Part model, mm, in its own coordinate system. Coordinates: 2 decimals unless noted, no trailing zeros. Loops run counter-clockwise (first coordinate to the right, second up) from the corner with the lowest first, then second, coordinate; pieces in that order, holes last. Notation, with made-up numbers: (-34, -34.5) -> (-3, -34.5) arc R8 cw to (-3, -26.5) -> close; hole circle Ø7 at (-11, 79.25). An arc over 180 degrees is marked (long way). One line per question, with ' | ' between items. Start each with the question number.
1) Cut at A-A (x = 75). List the corners of the cut face in (y, z), plus the area to 3 significant figures.
2) Cut at C-C (z = 53). List the corners of the cut face in (x, y).
3) Cut at B-B (z = -399.5). List the corners of the cut face in (x, y).
4) Probe L1, parallel to Y at x = 64, z = -62; L2, parallel to Y at x = 82, z = -1046. List the from-to ranges inside material, lowest first. Write a range as from..to.
5) Drop flat-ended pins along their axis: pin 1 (6 mm diameter, centred on x = 56.5, y = 4, fed in from -Z); pin 2 (8 mm diameter, centred on x = 34, z = 36, fed in from +Y); pin 3 (4 mm diameter, centred on x = 45, y = 24, fed in from -Z). Give the stop position or say it passes through.
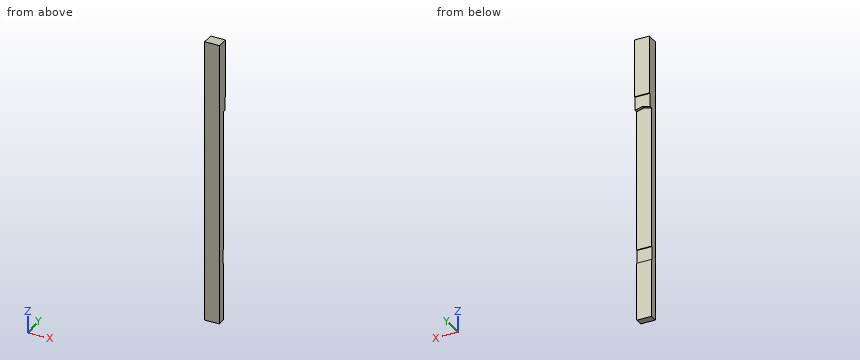
Autodesk Inventor part; units mm, degrees
ref_plane "YZ Plane" through (0, 0, 0) normal (1, 0, 0) x (0, 1, 0)
ref_plane "XZ Plane" through (0, 0, 0) normal (0, 1, 0) x (-1, 0, 0)
ref_plane "XY Plane" through (0, 0, 0) normal (0, 0, 1) x (1, 0, 0)
sketch "Эскиз1" plane through (0, 0, 0) normal (1, 0, 0) x (0, 1, 0)
  line L0 (0, 0) -> (0, -970)
  line L1 (0, -970) -> (-5, -970)
  line L2 (-5, -970) -> (-5, -1063)
  line L3 (-5, -1063) -> (0, -1063)
  line L4 (0, -1063) -> (0, -1463)
  line L5 (0, -1463) -> (-50, -1463)
  line L6 (-50, -1463) -> (-50, 493)
  line L7 (0, 0) -> (21, 0)
  line L8 (21, 0) -> (21, 93)
  line L9 (21, 93) -> (26, 93)
  line L10 (26, 93) -> (26, 493)
  line L11 (26, 493) -> (-50, 493)
  dimension "d0" = 970
  dimension "d1" = 5
  dimension "d2" = 93
  dimension "d3" = 400
  dimension "d4" = 50
  dimension "d5" = 21
  dimension "d6" = 93
  dimension "d7" = 5
  dimension "d8" = 400
  dimension "d9" = 1956
extrude "Выдавливание1" add sketch "Эскиз1" along normal blind 100
sketch "Эскиз2" plane through (0, 21, 93) normal (0, 1, 0) x (1, 0, 0)
  line L0 (0, 91.3764) -> (49.9516, 78.389)
  line L1 (0, 93) -> (0, 91.3764)
  line L2 (0, 93) -> (99.9032, 93)
  line L3 (99.9032, 91.3764) -> (99.9032, 93)
  line L4 (49.9516, 78.389) -> (99.9032, 91.3764)
extrude "Выдавливание2" cut sketch "Эскиз2" against normal up to surface (21 mm away)
properties part number "ground_all"
Reported:
1) outline: (-50, -1463) -> (0, -1463) -> (0, -1063) -> (-5, -1063) -> (-5, -970) -> (0, -970) -> (0, 8.1) -> (21, 8.1) -> (21, 93) -> (26, 93) -> (26, 493) -> (-50, 493) -> close | area: 110,000 mm²
2) outline: (0, -50) -> (100, -50) -> (100, 21) -> (0, 21) -> close
3) outline: (0, -50) -> (100, -50) -> (100, 0) -> (0, 0) -> close
4) L1: y = -50..0 | L2: y = -50..-5
5) pin 1: stops at z = 12.13 | pin 2: stops at y = 21 | pin 3: stops at z = 93
